Part print with two shaded views. Sizes in mm from the minimum x, y, z corner. A direction names the side the tool comes from. Coordinates: 2 decimals unless noted, no trailing zeros. Order: outer loops, then holes, each group sorted by start corner. A loop starts at its lowest first (then second) coordinate and runs counter-clockwise, first axis right, second up. Notation, with made-up numbers: (66.5, 1.25) - (101.5, 1.25) arc R24 ccw to (101.5, 28.25) - close; hole circle Ø10 at (85.5, 35). An arc over 180 degrees is marked (long way). One line per item, written item: value.
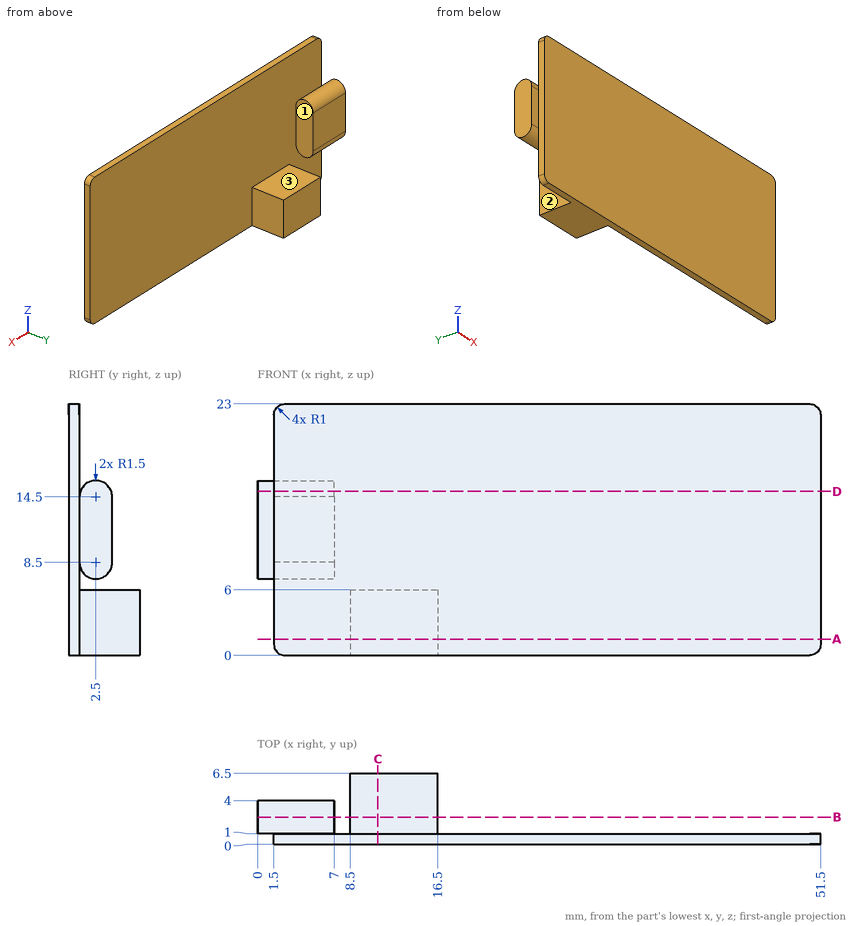
1. Band-saw the part on A-A, the plane z = 1.5. Give the cut face in (x, y), and give its area (3 significant figures).
Values found:
outline: (1.5, 0) - (51.5, 0) - (51.5, 1) - (16.5, 1) - (16.5, 6.5) - (8.5, 6.5) - (8.5, 1) - (1.5, 1) - close
area: 94.0 mm2
2. Flat gauge pins, fed straight in: P1, Ø5, axis at x = 3.5, z = 12, coming from the +Y side; P2, Ø4, axis at x = 9, z = 17, coming from the +Y side; P3, Ø0.8, axis at y = 0.5, z = 10.5, coming from the -X side. Where does each tip first touch, or does it go through?
Values found:
P1: stops at y = 4
P2: stops at y = 1
P3: stops at x = 1.5
3. Band-saw the part on B-B, the plane y = 2.5. Give the cut face in (x, z), and give its area (3 significant figures).
Values found:
outline: (0, 7) - (7, 7) - (7, 16) - (0, 16) - close; (8.5, 0) - (16.5, 0) - (16.5, 6) - (8.5, 6) - close
area: 111 mm2
4. Probe line 1 along Y through (x, z) = (17, 15.25); line 2 along X through (y, z) = (2.75, 5.75); line 3 along Z through (x, y) = (12.5, 2.75). List the from-to ranges inside material, lowest first.
Values found:
line 1: y = 0 to 1
line 2: x = 8.5 to 16.5
line 3: z = 0 to 6
5. 3-axis set-ups, long thin cutter, end or side, ignore diameter. For the marked faces 1, 2 and 3: which of +Z, -Z, +X, -X, +Y, -Y reach the whole face in a straight line?
Values found:
face 1: +Z, -Z, +X, +Y
face 2: +Z, -Z, -X, +Y
face 3: +Z, +X, -X, +Y
6. Band-saw the part on D-D, the plane z = 15. Give the cut face in (x, y), and give its area (3 significant figures).
Values found:
outline: (0, 1.09) - (7, 1.09) - (7, 3.91) - (0, 3.91) - close; (1.5, 0) - (51.5, 0) - (51.5, 1) - (1.5, 1) - close
area: 69.8 mm2
7. Band-saw the part on C-C, the plane x = 11. Give the cut face in (y, z).
Values found:
outline: (0, 0) - (6.5, 0) - (6.5, 6) - (1, 6) - (1, 23) - (0, 23) - close
